The listing builds one solid part. Answer for the finished solid, in the listing's coordinates (mm). Face numbers are marked on the shaded views. A direction names the side the tool comes from. Give positions to 0.01 mm unless a question says otherwise; leave off trailing zeros. Order: outer loops, then holes, each group sorted by start corner. A loop starts at its lowest first (then second) coordinate and runs counter-clockwise, first axis right, second up. Notation, with made-up numbers: (-23, -24.5) - (28, -24.5) arc R26 cw to (28, 13.5) - close; hole circle Ø2 at (-0.75, 39). An arc over 180 degrees is marked (long way). Answer as CSV lines item,"result". Start each with the question number.
1. Consider line 1 along Y through (x, z) = (11.9, 9.1) (3 decimals); line 2 along X through (y, z) = (3.9, 9.2) (3 decimals); line 3 along Y through (x, z) = (15.9, 5.75). Determine where each line is inside the solid, lowest interval first. Write a range as [from, to].
2. Flat-ended cylindrical pins translate along their axes: pin 1 (6 mm diameter, centred on x = 28.5, y = 4, fed in from -Z); pin 2 (1.9 mm diameter, centred on x = 27.9, y = 3.9, fed in from -Z); pin 3 (2.5 mm diameter, centred on x = 19.9, y = 11.9, fed in from -Z); pin 4 (4.5 mm diameter, centred on x = 23.9, y = 7.9, fed in from +Z). Find the tip coordinate at first contact, or state that the pin passes through.
3. Section A-A on z = 7.75 is taken. Give the vertices of the cut face in (x, y).
4. Section C-C on x = 15.9 is taken. Give the vertices of the cut face in (y, z).
5. Section D-D on x = 27.9 is taken. Give the vertices of the cut face in (y, z) (3 decimals), and give its area (3 significant figures).
6. Determine the mould class of the marked faces 4, 5 and 6 for opening direction Y: +Y half, -Y half, draft (parallel to the pull), parting line (faces both ways), or undercut.
7. Which of the six approach directions +Z, -Z, +X, -X, +Y, -Y give full straight-line access (tool end or side, diameter ignored) to the marked faces 1, 2 and 3?
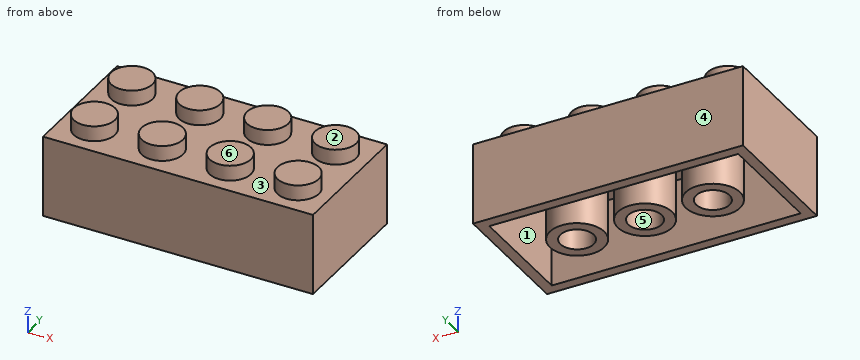
from build123d import *

# Parameters (mm, degrees)
F0_W        = 31.8
F0_H        = 15.8
F1_DEPTH    = 9.6
F2_R        = 2.435
F3_DEPTH    = 1.8
F4_T        = -1.24
F5_R        = 3.2
F6_DEPTH    = 8.36
F7_T        = 1.24
F7_T3_DEPTH = 10.84
F7_T5_DEPTH = 15.8
F7_T7_DEPTH = 31.8


# Not quite as in the source:
# - a shell that OpenCascade refuses in one call is made with other operations: the cavity is built on its own and cut out


with BuildPart() as f1:
    # F0 (on Top) → F1 (new body)
    with BuildSketch(Plane.XY):
        with Locations((15.9, 7.9)):
            Rectangle(F0_W, F0_H)
    extrude(amount=F1_DEPTH)

    # F2 (on face) → F3 (join)
    with BuildSketch(Plane.XY.offset(9.6)):
        with Locations((3.9, 11.9)):
            Circle(F2_R)
        with Locations((11.9, 11.9)):
            Circle(F2_R)
        with Locations((19.9, 11.9)):
            Circle(F2_R)
        with Locations((27.9, 11.9)):
            Circle(F2_R)
        with Locations((27.9, 3.9)):
            Circle(F2_R)
        with Locations((19.9, 3.9)):
            Circle(F2_R)
        with Locations((11.9, 3.9)):
            Circle(F2_R)
        with Locations((3.9, 3.9)):
            Circle(F2_R)
    extrude(amount=F3_DEPTH)

    # F4
    f4_openings = [f1.faces().sort_by_distance(p)[0] for p in [
        (15.9, 7.9, 0),
    ]]
    offset(amount=F4_T, openings=f4_openings, kind=Kind.INTERSECTION)

    # F5 (on face) → F6 (join)
    with BuildSketch(Plane(origin=(0, 0, 8.36), x_dir=(1, 0, 0), z_dir=(0, 0, -1))):
        with Locations((7.9, -7.9)):
            Circle(F5_R)
        with Locations((15.9, -7.9)):
            Circle(F5_R)
        with Locations((23.9, -7.9)):
            Circle(F5_R)
    extrude(amount=F6_DEPTH)

    # F7: shell of thickness 1.24, made by hand


with BuildPart() as f7_core1:
    # F7_t2: copy of F1
    add(f1.part)

    # the walls: a layer under each face that stays
    f7_faces = [f7_core1.faces().sort_by_distance(p)[0] for p in [
        (0, 7.9, 4.8),
        (15.9, 15.8, 4.8),
        (15.9, 0, 4.8),
        (2.2714285714, 1.1285714286, 0),
        (15.9, 7.9, 9.6),
        (31.8, 7.9, 4.8),
        (1.24, 7.9, 4.18),
        (15.9, 14.56, 4.18),
        (30.56, 7.9, 4.18),
        (15.9, 1.24, 4.18),
        (1.465, 3.9, 10.5),
        (9.465, 3.9, 10.5),
        (17.465, 3.9, 10.5),
        (25.465, 3.9, 10.5),
        (1.465, 11.9, 10.5),
        (9.465, 11.9, 10.5),
        (17.465, 11.9, 10.5),
        (25.465, 11.9, 10.5),
        (6.1266666667, 3.46, 8.36),
        (3.9, 3.9, 11.4),
        (11.9, 3.9, 11.4),
        (19.9, 3.9, 11.4),
        (27.9, 3.9, 11.4),
        (3.9, 11.9, 11.4),
        (11.9, 11.9, 11.4),
        (19.9, 11.9, 11.4),
        (27.9, 11.9, 11.4),
        (2.705, 3.9, 9.26),
        (10.705, 3.9, 9.26),
        (18.705, 3.9, 9.26),
        (26.705, 3.9, 9.26),
        (4.7, 7.9, 4.18),
        (2.705, 11.9, 9.26),
        (10.705, 11.9, 9.26),
        (12.7, 7.9, 4.18),
        (20.7, 7.9, 4.18),
        (18.705, 11.9, 9.26),
        (26.705, 11.9, 9.26),
        (3.9, 3.9, 10.16),
        (11.9, 3.9, 10.16),
        (19.9, 3.9, 10.16),
        (27.9, 3.9, 10.16),
        (3.9, 11.9, 10.16),
        (11.9, 11.9, 10.16),
        (19.9, 11.9, 10.16),
        (27.9, 11.9, 10.16),
    ]]
    thicken(f7_faces, amount=-F7_T, mode=Mode.SUBTRACT)

    # F7_s4 → F7_t3 (cut)
    with BuildSketch(Plane.XY.offset(-1.24)):
        Polygon((1.2524, 14.5476), (0, 14.56), (0, 15.8), (1.24, 15.8), align=None)
        Polygon((1.2524, 1.2524), (0, 1.24), (0, 0), (1.24, 0), align=None)
        Polygon((30.5476, 14.5476), (30.56, 15.8), (31.8, 15.8), (31.8, 14.56), align=None)
        Polygon((30.5476, 1.2524), (31.8, 1.24), (31.8, 0), (30.56, 0), align=None)
    extrude(amount=F7_T3_DEPTH, mode=Mode.SUBTRACT)

    # F7_s6 → F7_t5 (cut)
    with BuildSketch(Plane.XZ.offset(-15.8)):
        Polygon((1.2524, 8.3476), (0, 8.36), (0, 9.6), (1.24, 9.6), align=None)
        Polygon((30.5476, 8.3476), (31.8, 8.36), (31.8, 9.6), (30.56, 9.6), align=None)
    extrude(amount=F7_T5_DEPTH, mode=Mode.SUBTRACT)

    # F7_s8 → F7_t7 (cut)
    with BuildSketch(Plane.YZ):
        Polygon((14.5476, 8.3476), (15.8, 8.36), (15.8, 9.6), (14.56, 9.6), align=None)
        Polygon((1.2524, 8.3476), (0, 8.36), (0, 9.6), (1.24, 9.6), align=None)
    extrude(amount=F7_T7_DEPTH, mode=Mode.SUBTRACT)

    # F7_s9 → F7_t10 (revolve, cut)
    with BuildSketch(Plane.XZ.offset(-3.9)):
        Polygon((6.3474, 9.6124), (6.335, 8.36), (5.095, 8.36), (5.095, 9.6), align=None)
    revolve(axis=Axis((3.9, 3.9, 9.6), (0, 0, 1)), mode=Mode.SUBTRACT)

    # F7_s11 → F7_t12 (revolve, cut)
    with BuildSketch(Plane.XZ.offset(-3.9)):
        Polygon((14.3474, 9.6124), (14.335, 8.36), (13.095, 8.36), (13.095, 9.6), align=None)
    revolve(axis=Axis((11.9, 3.9, 9.6), (0, 0, 1)), mode=Mode.SUBTRACT)

    # F7_s13 → F7_t14 (revolve, cut)
    with BuildSketch(Plane.XZ.offset(-3.9)):
        Polygon((22.3474, 9.6124), (22.335, 8.36), (21.095, 8.36), (21.095, 9.6), align=None)
    revolve(axis=Axis((19.9, 3.9, 9.6), (0, 0, 1)), mode=Mode.SUBTRACT)

    # F7_s15 → F7_t16 (revolve, cut)
    with BuildSketch(Plane.XZ.offset(-3.9)):
        Polygon((30.3474, 9.6124), (30.335, 8.36), (29.095, 8.36), (29.095, 9.6), align=None)
    revolve(axis=Axis((27.9, 3.9, 9.6), (0, 0, 1)), mode=Mode.SUBTRACT)

    # F7_s17 → F7_t18 (revolve, cut)
    with BuildSketch(Plane.XZ.offset(-11.9)):
        Polygon((6.3474, 9.6124), (6.335, 8.36), (5.095, 8.36), (5.095, 9.6), align=None)
    revolve(axis=Axis((3.9, 11.9, 9.6), (0, 0, 1)), mode=Mode.SUBTRACT)

    # F7_s19 → F7_t20 (revolve, cut)
    with BuildSketch(Plane.XZ.offset(-11.9)):
        Polygon((14.3474, 9.6124), (14.335, 8.36), (13.095, 8.36), (13.095, 9.6), align=None)
    revolve(axis=Axis((11.9, 11.9, 9.6), (0, 0, 1)), mode=Mode.SUBTRACT)

    # F7_s21 → F7_t22 (revolve, cut)
    with BuildSketch(Plane.XZ.offset(-11.9)):
        Polygon((22.3474, 9.6124), (22.335, 8.36), (21.095, 8.36), (21.095, 9.6), align=None)
    revolve(axis=Axis((19.9, 11.9, 9.6), (0, 0, 1)), mode=Mode.SUBTRACT)

    # F7_s23 → F7_t24 (revolve, cut)
    with BuildSketch(Plane.XZ.offset(-11.9)):
        Polygon((30.3474, 9.6124), (30.335, 8.36), (29.095, 8.36), (29.095, 9.6), align=None)
    revolve(axis=Axis((27.9, 11.9, 9.6), (0, 0, 1)), mode=Mode.SUBTRACT)

    # F7_s25 → F7_t26 (revolve, cut)
    with BuildSketch(Plane.XZ.offset(-7.9)):
        Polygon((11.1124, 8.3476), (11.1, 9.6), (9.86, 9.6), (9.86, 8.36), align=None)
    revolve(axis=Axis((7.9, 7.9, 8.36), (0, 0, -1)), mode=Mode.SUBTRACT)

    # F7_s27 → F7_t28 (revolve, cut)
    with BuildSketch(Plane.XZ.offset(-7.9)):
        Polygon((19.1124, 8.3476), (19.1, 9.6), (17.86, 9.6), (17.86, 8.36), align=None)
    revolve(axis=Axis((15.9, 7.9, 8.36), (0, 0, -1)), mode=Mode.SUBTRACT)

    # F7_s29 → F7_t30 (revolve, cut)
    with BuildSketch(Plane.XZ.offset(-7.9)):
        Polygon((27.1124, 8.3476), (27.1, 9.6), (25.86, 9.6), (25.86, 8.36), align=None)
    revolve(axis=Axis((23.9, 7.9, 8.36), (0, 0, -1)), mode=Mode.SUBTRACT)

    # F7_s31 → F7_t32 (revolve, cut)
    with BuildSketch(Plane.XZ.offset(-3.9)):
        Polygon((5.0826, 10.1476), (6.335, 10.16), (6.335, 11.4), (5.095, 11.4), align=None)
    revolve(axis=Axis((3.9, 3.9, 10.16), (0, 0, -1)), mode=Mode.SUBTRACT)

    # F7_s33 → F7_t34 (revolve, cut)
    with BuildSketch(Plane.XZ.offset(-3.9)):
        Polygon((13.0826, 10.1476), (14.335, 10.16), (14.335, 11.4), (13.095, 11.4), align=None)
    revolve(axis=Axis((11.9, 3.9, 10.16), (0, 0, -1)), mode=Mode.SUBTRACT)

    # F7_s35 → F7_t36 (revolve, cut)
    with BuildSketch(Plane.XZ.offset(-3.9)):
        Polygon((21.0826, 10.1476), (22.335, 10.16), (22.335, 11.4), (21.095, 11.4), align=None)
    revolve(axis=Axis((19.9, 3.9, 10.16), (0, 0, -1)), mode=Mode.SUBTRACT)

    # F7_s37 → F7_t38 (revolve, cut)
    with BuildSketch(Plane.XZ.offset(-3.9)):
        Polygon((29.0826, 10.1476), (30.335, 10.16), (30.335, 11.4), (29.095, 11.4), align=None)
    revolve(axis=Axis((27.9, 3.9, 10.16), (0, 0, -1)), mode=Mode.SUBTRACT)

    # F7_s39 → F7_t40 (revolve, cut)
    with BuildSketch(Plane.XZ.offset(-11.9)):
        Polygon((5.0826, 10.1476), (6.335, 10.16), (6.335, 11.4), (5.095, 11.4), align=None)
    revolve(axis=Axis((3.9, 11.9, 10.16), (0, 0, -1)), mode=Mode.SUBTRACT)

    # F7_s41 → F7_t42 (revolve, cut)
    with BuildSketch(Plane.XZ.offset(-11.9)):
        Polygon((13.0826, 10.1476), (14.335, 10.16), (14.335, 11.4), (13.095, 11.4), align=None)
    revolve(axis=Axis((11.9, 11.9, 10.16), (0, 0, -1)), mode=Mode.SUBTRACT)

    # F7_s43 → F7_t44 (revolve, cut)
    with BuildSketch(Plane.XZ.offset(-11.9)):
        Polygon((21.0826, 10.1476), (22.335, 10.16), (22.335, 11.4), (21.095, 11.4), align=None)
    revolve(axis=Axis((19.9, 11.9, 10.16), (0, 0, -1)), mode=Mode.SUBTRACT)

    # F7_s45 → F7_t46 (revolve, cut)
    with BuildSketch(Plane.XZ.offset(-11.9)):
        Polygon((29.0826, 10.1476), (30.335, 10.16), (30.335, 11.4), (29.095, 11.4), align=None)
    revolve(axis=Axis((27.9, 11.9, 10.16), (0, 0, -1)), mode=Mode.SUBTRACT)


with BuildPart() as f1_1:
    add(f1.part)

    # what is left inside the walls is the cavity
    f7_cavity = [f7_core1.part.solids().sort_by_distance(p)[0] for p in [
        (5.9524, 7.9, 2.786667),
        (13.9524, 7.9, 2.786667),
        (21.9524, 7.9, 2.786667),
    ]]
    add(f7_cavity, mode=Mode.SUBTRACT)


solid = f1_1.part
Checks:
1,line 1,"y = [0, 2.705], [5.095, 10.705], [13.095, 15.8]"
1,line 2,"x = [0, 2.705], [5.095, 10.705], [13.095, 18.705], [21.095, 26.705], [29.095, 31.8]"
1,line 3,"y = [0, 1.24], [4.7, 5.94], [9.86, 11.1], [14.56, 15.8]"
2,pin 1,"stops at z = 0"
2,pin 2,"stops at z = 10.16"
2,pin 3,"stops at z = 8.36"
2,pin 4,"stops at z = 9.6"
3,outline,"(0, 0) - (31.8, 0) - (31.8, 15.8) - (0, 15.8) - close; circle Ø6.4 at (7.9, 7.9); circle Ø6.4 at (15.9, 7.9); circle Ø6.4 at (23.9, 7.9); hole (1.24, 1.24) - (30.56, 1.24) - (30.56, 14.56) - (1.24, 14.56) - close; hole circle Ø3.92 at (7.9, 7.9); hole circle Ø3.92 at (15.9, 7.9); hole circle Ø3.92 at (23.9, 7.9)"
4,outline,"(0, 0) - (1.24, 0) - (1.24, 8.36) - (4.7, 8.36) - (4.7, 0) - (5.94, 0) - (5.94, 8.36) - (9.86, 8.36) - (9.86, 0) - (11.1, 0) - (11.1, 8.36) - (14.56, 8.36) - (14.56, 0) - (15.8, 0) - (15.8, 9.6) - (0, 9.6) - close"
5,outline,"(0, 0) - (1.24, 0) - (1.24, 8.36) - (2.705, 8.36) - (2.705, 10.16) - (5.095, 10.16) - (5.095, 8.36) - (10.705, 8.36) - (10.705, 10.16) - (13.095, 10.16) - (13.095, 8.36) - (14.56, 8.36) - (14.56, 0) - (15.8, 0) - (15.8, 9.6) - (14.335, 9.6) - (14.335, 11.4) - (9.465, 11.4) - (9.465, 9.6) - (6.335, 9.6) - (6.335, 11.4) - (1.465, 11.4) - (1.465, 9.6) - (0, 9.6) - close"
5,area,"49.3 mm²"
6,face 4,"+Y half"
6,face 5,"undercut"
6,face 6,"draft"
7,face 1,"-Z"
7,face 2,"+Z, +X, -X, +Y, -Y"
7,face 3,"+Z"
